Here's how the part is built. I have some questions about the finished solid (model axes, mm). Face numbers are marked on the shaded views. A direction names the side the tool comes from. Round coordinates to 2 decimals unless told otherwise and drop trailing zeros. Loops run counter-clockwise (first coordinate to the right, second up) from the corner with the lowest first, then second, coordinate; pieces in that order, holes last. Notation, with made-up numbers: M 61,21 L 74,21 A6 ccw 74,30 Z; hole C 4.25,29 d10. An arc over 180 degrees is marked long. Answer as a JSON object with one key per item and string values.
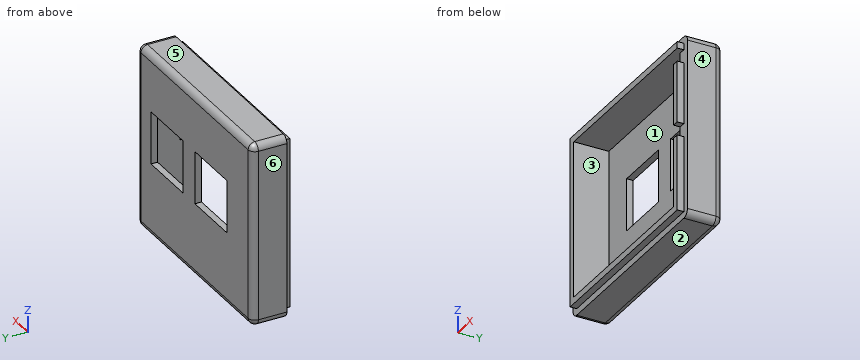
from build123d import *

# Parameters (mm, degrees)
SKETCH1_W           = 95
SKETCH1_H           = 83.5
SKETCH1_W_2         = 89
SKETCH1_H_2         = 77.5
SKETCH1_W_3         = 83
SKETCH1_H_3         = 71.5
BOSS_EXTRUDE1_DEPTH = 3
SKETCH1_4_W         = 95
SKETCH1_4_H         = 83.5
SKETCH1_4_W_2       = 89
SKETCH1_4_H_2       = 77.5
SKETCH1_4_W_3       = 83
SKETCH1_4_H_3       = 71.5
BOSS_EXTRUDE2_DEPTH = 16
SKETCH1_5_W         = 89
SKETCH1_5_H         = 77.5
SKETCH1_5_W_2       = 83
SKETCH1_5_H_2       = 71.5
BOSS_EXTRUDE3_DEPTH = 19
FILLET1_R           = 3
SKETCH3_W           = 6
SKETCH3_H           = 6
CUT_EXTRUDE1_DEPTH  = 6
CUT_EXTRUDE2_REACH  = 5
SKETCH4_W           = 26.5
SKETCH4_H           = 24


with BuildPart() as part:
    # Sketch1 → Boss-Extrude1 (new body)
    with BuildSketch(Plane(origin=(0, 0, 0), x_dir=(1, 0, 0), z_dir=(0, 1, 0))):
        Rectangle(SKETCH1_W, SKETCH1_H)
        Rectangle(SKETCH1_W_2, SKETCH1_H_2, mode=Mode.SUBTRACT)
        Rectangle(SKETCH1_W_2, SKETCH1_H_2)
        Rectangle(SKETCH1_W_3, SKETCH1_H_3, mode=Mode.SUBTRACT)
        Rectangle(SKETCH1_W_3, SKETCH1_H_3)
    extrude(amount=-BOSS_EXTRUDE1_DEPTH)

    # Sketch1_4 → Boss-Extrude2 (add)
    with BuildSketch(Plane(origin=(0, 0, 0), x_dir=(1, 0, 0), z_dir=(0, 1, 0))):
        Rectangle(SKETCH1_4_W, SKETCH1_4_H)
        Rectangle(SKETCH1_4_W_2, SKETCH1_4_H_2, mode=Mode.SUBTRACT)
        Rectangle(SKETCH1_4_W_2, SKETCH1_4_H_2)
        Rectangle(SKETCH1_4_W_3, SKETCH1_4_H_3, mode=Mode.SUBTRACT)
    extrude(amount=-BOSS_EXTRUDE2_DEPTH)

    # Sketch1_5 → Boss-Extrude3 (add)
    with BuildSketch(Plane(origin=(0, 0, 0), x_dir=(1, 0, 0), z_dir=(0, 1, 0))):
        Rectangle(SKETCH1_5_W, SKETCH1_5_H)
        Rectangle(SKETCH1_5_W_2, SKETCH1_5_H_2, mode=Mode.SUBTRACT)
    extrude(amount=-BOSS_EXTRUDE3_DEPTH)

    # Fillet1
    fillet1_edges = [part.edges().sort_by_distance(p)[0] for p in [
        (-47.5, 0, 0),
        (0, 0, -41.75),
        (47.5, 0, 0),
        (0, 0, 41.75),
        (-47.5, -8, 41.75),
        (-47.5, -8, -41.75),
        (47.5, -8, -41.75),
        (47.5, -8, 41.75),
    ]]
    fillet(fillet1_edges, radius=FILLET1_R)

    # Sketch3 → Cut-Extrude1 (cut)
    with BuildSketch(Plane(origin=(47.5, 0, 0), x_dir=(0, 0, -1), z_dir=(1, 0, 0))):
        with Locations((-32.75, -19)):
            Rectangle(SKETCH3_W, SKETCH3_H)
        with Locations((1.25, -19)):
            Rectangle(SKETCH3_W, SKETCH3_H)
    extrude(amount=-CUT_EXTRUDE1_DEPTH, mode=Mode.SUBTRACT)

    # Sketch4 → Cut-Extrude2 (cut, up to next)
    with BuildSketch(Plane.XZ.offset(3), mode=Mode.PRIVATE) as cut_extrude2_sk1:
        with Locations((-13.5, 3.75)):
            Rectangle(SKETCH4_W, SKETCH4_H)
    cut_extrude2_tool1 = extrude(cut_extrude2_sk1.sketch, amount=-CUT_EXTRUDE2_REACH, mode=Mode.PRIVATE) & part.part
    add(cut_extrude2_tool1.solids().sort_by_distance((-13.5, -3, 3.75))[0], mode=Mode.SUBTRACT)
    # Sketch4 → Cut-Extrude2 (cut, up to next)
    with BuildSketch(Plane.XZ.offset(3), mode=Mode.PRIVATE) as cut_extrude2_sk2:
        with Locations((23, 3.75)):
            Rectangle(SKETCH4_W, SKETCH4_H)
    cut_extrude2_tool2 = extrude(cut_extrude2_sk2.sketch, amount=-CUT_EXTRUDE2_REACH, mode=Mode.PRIVATE) & part.part
    add(cut_extrude2_tool2.solids().sort_by_distance((23, -3, 3.75))[0], mode=Mode.SUBTRACT)


solid = part.part
Item 1: I want a section at D-D on x = -33. List the corners of the cut face in (y, z) for me.
Solution:
{"outline": "M -19,-38.75 L -16,-38.75 L -16,-41.75 L -3,-41.75 A3 ccw 0,-38.75 L 0,38.75 A3 ccw -3,41.75 L -16,41.75 L -16,38.75 L -19,38.75 L -19,35.75 L -3,35.75 L -3,-35.75 L -19,-35.75 Z"}
Item 2: We'd pull the mould along X, two halves only. Please class the marked faces 3, 4, 5 and 6: +X half, -X half, draft (parallel to the pull), parting line (faces both ways), or undercut.
Solution:
{"face 3": "undercut", "face 4": "+X half", "face 5": "draft", "face 6": "-X half"}
Item 3: For the marked faces 1 and 2, which set-ups out of +Z, -Z, +X, -X, +Y, -Y let a thin tool reach every point of the face, with its end or its side?
Solution:
{"face 1": "-Y", "face 2": "-Z, +X, -X, +Y, -Y"}
Item 4: I want a section at C-C on y = -11. List the corners of the cut face in (x, z) for me, plus the area to 3 significant figures.
Solution:
{"outline": "M -47.5,-38.75 A3 ccw -44.5,-41.75 L 44.5,-41.75 A3 ccw 47.5,-38.75 L 47.5,38.75 A3 ccw 44.5,41.75 L -44.5,41.75 A3 ccw -47.5,38.75 Z; hole M -41.5,-35.75 L 41.5,-35.75 L 41.5,35.75 L -41.5,35.75 Z", "area": "1,990 mm2"}
Item 5: If I drill on L1, parallel to X at y = -17.75, z = 8; L2, parallel to Z at x = 15.5, y = -13; L3, parallel to X at y = -14.5, z = 34, over which ranges is the centre line in solid material (lowest first)? Write a range as from..to.
Solution:
{"L1": "x = -44.5..-41.5, 41.5..44.5", "L2": "z = -41.75..-35.75, 35.75..41.75", "L3": "x = -47.5..-41.5, 41.5..47.5"}
Item 6: I want a section at A-A on x = 19. List the corners of the cut face in (y, z) for me, plus the area to 3 significant figures.
Solution:
{"outline": "M -19,-38.75 L -16,-38.75 L -16,-41.75 L -3,-41.75 A3 ccw 0,-38.75 L 0,-8.25 L -3,-8.25 L -3,-35.75 L -19,-35.75 Z; M -19,35.75 L -3,35.75 L -3,15.75 L 0,15.75 L 0,38.75 A3 ccw -3,41.75 L -16,41.75 L -16,38.75 L -19,38.75 Z", "area": "349 mm2"}
Item 7: I want a section at B-B on z = 0. List the corners of the cut face in (x, y) for me.
Solution:
{"outline": "M -47.5,-16 L -44.5,-16 L -44.5,-19 L -41.5,-19 L -41.5,-3 L -26.75,-3 L -26.75,0 L -44.5,0 A3 ccw -47.5,-3 Z; M -0.25,-3 L 9.75,-3 L 9.75,0 L -0.25,0 Z; M 36.25,-3 L 41.5,-3 L 41.5,-16 L 47.5,-16 L 47.5,-3 A3 ccw 44.5,0 L 36.25,0 Z"}
Item 8: For P1, Ø0.9, axis at x = 43, y = -17.5, coming from the -Z side; P2, Ø3.5, axis at y = -18, z = -13.5, coming from the -X side; P3, Ø3.5, axis at y = -1, z = 0.5, coming from the +X side, each with a flat end and sliding along its axis, tell me the tip position at first contact or that it passes through.
Solution:
{"P1": "stops at z = -38.75", "P2": "stops at x = -44.5", "P3": "stops at x = 47.49"}
